Could you check a few things on this model? Use its own coordinates, in mm. A direction names the side the tool comes from. Round coordinates to 2 decimals unless told otherwise and drop trailing zeros. Write each loop counter-clockwise with the first axis right and the second up, starting at its lowest first coordinate (ties: lowest second). Pieces come first, ordered by that corner, then holes. Notation, with made-up numbers: (29, -40) -> (47, -40) arc R20 ccw to (47, -6) -> close; hole circle Ø8 at (0, 36.5). An arc over 180 degrees is marked (long way). Return JSON: item names as keys, results as strings.
from build123d import *

# Parameters (mm, degrees)
CROQUIS1_W                          = 96
CROQUIS1_H                          = 55
SALIENTE_EXTRUIR2_DEPTH             = 15
CORTAR_EXTRUIR1_DEPTH               = 96
CORTAR_EXTRUIR6_REACH               = 17.673
CORTAR_EXTRUIR6_OFFSET_FROM_SURFACE = 1
CROQUIS4_W                          = 94
CROQUIS4_H                          = 54.224485051
CROQUIS5_R                          = 2
CORTAR_EXTRUIR7_DEPTH               = 97


with BuildPart() as part:
    # Croquis1 → Saliente-Extruir2 (new body)
    with BuildSketch(Plane.XY):
        Rectangle(CROQUIS1_W, CROQUIS1_H)
    extrude(amount=SALIENTE_EXTRUIR2_DEPTH)

    # Croquis2 → Cortar-Extruir1 (cut)
    with BuildSketch(Plane.ZY.offset(48)):
        Polygon((3.329836367, 27.5), (15, 27.5), (15, -27.5), align=None)
    extrude(amount=-CORTAR_EXTRUIR1_DEPTH, mode=Mode.SUBTRACT)

    # Cortar-Extruir6: up to this face of the body (flat: up to its plane, moved by the offset)
    cortar_extruir6_end = Plane(part.part.faces().sort_by_distance((0, 0, 0))[0]).offset(-CORTAR_EXTRUIR6_OFFSET_FROM_SURFACE)
    # Croquis4 → Cortar-Extruir6 (cut, up to the picked face)
    with BuildSketch(Plane(origin=(0, 1.860875227, 8.770068758), x_dir=(1, 0, 0), z_dir=(0, 0.207563726, 0.978221498)), mode=Mode.PRIVATE) as cortar_extruir6_sk1:
        with Locations((0, -1.902304571)):
            Rectangle(CROQUIS4_W, CROQUIS4_H)
    cortar_extruir6_tool1 = split(extrude(cortar_extruir6_sk1.sketch, amount=-CORTAR_EXTRUIR6_REACH, mode=Mode.PRIVATE), bisect_by=cortar_extruir6_end, keep=Keep.BOTH, mode=Mode.PRIVATE)
    add(cortar_extruir6_tool1.solids().sort_by_distance((0, 0, 9.164918))[0], mode=Mode.SUBTRACT)

    # Croquis5 → Cortar-Extruir7 (cut, through all)
    with BuildSketch(Plane.ZY.offset(48)):
        with Locations((4.526520959, -21.5)):
            Circle(CROQUIS5_R)
    extrude(amount=-CORTAR_EXTRUIR7_DEPTH, mode=Mode.SUBTRACT)


solid = part.part
1) For faces 4 (the face through (-48, -6, 6)), 5 (the face through (-0.658, -27.004, 12.52)), which set-ups out of +Z, -Z, +X, -X, +Y, -Y let a thin tool reach every point of the face, with its end or its side?
Return value:
{"face 4": "+Z, -Z, -X, +Y, -Y", "face 5": "+Y"}
2) I want a section at A-A, the plane y = -21.5. Please give me the cut outline in (x, z), and give its area (3 significant figures).
Return value:
{"outline": "(-48, 0) -> (48, 0) -> (48, 2.53) -> (47, 2.53) -> (47, 1) -> (-47, 1) -> (-47, 2.53) -> (-48, 2.53) -> close; (-48, 6.53) -> (-47, 6.53) -> (-47, 13.73) -> (-48, 13.73) -> close; (47, 6.53) -> (48, 6.53) -> (48, 13.73) -> (47, 13.73) -> close", "area": "113 mm²"}
3) Thinking about a two-plate mould opening in Z: for faces 1 (the face through (-47.507, -19.517, 4.266)), 2 (the face through (-1, -27.5, 11)), 3 (the face through (-0.658, 26.256, 2.286)), which applies, pulls with the +Z half, pulls with the -Z half, needs draft (parallel to the pull), parting line crosses it, or undercut?
Return value:
{"face 1": "undercut", "face 2": "needs draft", "face 3": "pulls with the +Z half"}
4) I want a section at D-D, the plane y = -4.5. Please give me the cut outline in (x, z), and give its area (3 significant figures).
Return value:
{"outline": "(-48, 0) -> (48, 0) -> (48, 10.12) -> (47, 10.12) -> (47, 1) -> (-47, 1) -> (-47, 10.12) -> (-48, 10.12) -> close", "area": "114 mm²"}
5) Will these pins go through, and if not, where does the flat tip stop? pin 1 Ø3.5 at (y, z) = (-21.5, 4.53) entering from +X; pin 2 Ø4.5 at (y, z) = (-21.5, 4.53) entering from -X; pin 3 Ø12 at (x, y) = (12.5, -1) entering from +Z.
Return value:
{"pin 1": "through", "pin 2": "x = -48", "pin 3": "z = 1"}
6) I want a section at B-B, the plane x = 39.5. Please give me the cut outline in (y, z).
Return value:
{"outline": "(-27.5, 0) -> (27.5, 0) -> (27.5, 3.33) -> (26.52, 3.54) -> (25.98, 1) -> (-27.5, 1) -> close; (-27.5, 10.18) -> (-26.52, 14.79) -> (-27.5, 15) -> close"}
7) If I drill on probe 1 along X at (y, z) = (2.5, 4.25); probe 2 along Z at (x, y) = (38.5, 9.5); probe 3 along Y at (x, z) = (-16.5, 2.25), over which ranges is the centre line in solid material (lowest first)? Write a range as [from, to].
Return value:
{"probe 1": "[-48, -47], [47, 48]", "probe 2": "[0, 1]", "probe 3": "[26.25, 27.5]"}
8) I want a section at C-C, the plane z = 7.75. Please give me the cut outline in (x, y), and give its area (3 significant figures).
Return value:
{"outline": "(-48, -27.5) -> (-47, -27.5) -> (-47, 6.67) -> (-48, 6.67) -> close; (47, -27.5) -> (48, -27.5) -> (48, 6.67) -> (47, 6.67) -> close", "area": "68.3 mm²"}
